```python
from build123d import *

# Parameters (mm, degrees)
EXTRUDE_1_DEPTH     = 15
SKETCH_2_R          = 22.25
EXTRUDE_2_DEPTH     = 560
SKETCH_3_R          = 20
EXTRUDE_3_DEPTH     = 25
SKETCH_4_R          = 4
CUT_EXTRUDE_4_DEPTH = 606.548993339
FILLET_1_R          = 1


with BuildPart() as part:
    # 草图1 → 拉伸1 (new body)
    with BuildSketch(Plane.XY):
        Polygon((37.527767497, 0), (18.763883749, 32.5), (-18.763883749, 32.5), (-37.527767497, 0), (-18.763883749, -32.5), (18.763883749, -32.5), align=None)
    extrude(amount=EXTRUDE_1_DEPTH)

    # 草图2 → 拉伸2 (add)
    with BuildSketch(Plane.XY.offset(15)):
        Circle(SKETCH_2_R)
    extrude(amount=EXTRUDE_2_DEPTH)

    # 草图3 → 拉伸3 (add)
    with BuildSketch(Plane.XY.offset(575)):
        Circle(SKETCH_3_R)
    extrude(amount=EXTRUDE_3_DEPTH)

    # 草图4 → 拉伸4 (cut, through all)
    with BuildSketch(Plane(origin=(-28.145825623, -16.25, 0), x_dir=(0, 0, 1), z_dir=(-0.8660254037844388, -0.4999999999999997, 0))):
        with Locations(Location((587.5, 0, 0), (0, 0, 270))):
            Circle(SKETCH_4_R)
    extrude(amount=-CUT_EXTRUDE_4_DEPTH, mode=Mode.SUBTRACT)

    # 圆角1
    fillet_1_edges = [part.edges().sort_by_distance(p)[0] for p in [
        (0, 32.5, 15),
        (-28.145825623, 16.25, 15),
        (-28.145825623, -16.25, 15),
        (0, -32.5, 15),
        (-22.25, 0, 575),
        (-20, 0, 600),
        (-18.970562748, -6.333857356, 587.5),
        (14.970562748, 13.262060586, 587.5),
        (28.145825623, -16.25, 15),
        (0, -32.5, 0),
        (-28.145825623, -16.25, 0),
        (-28.145825623, 16.25, 0),
        (28.145825623, 16.25, 15),
        (0, 32.5, 0),
        (28.145825623, 16.25, 0),
        (28.145825623, -16.25, 0),
    ]]
    fillet(fillet_1_edges, radius=FILLET_1_R)


solid = part.part
```
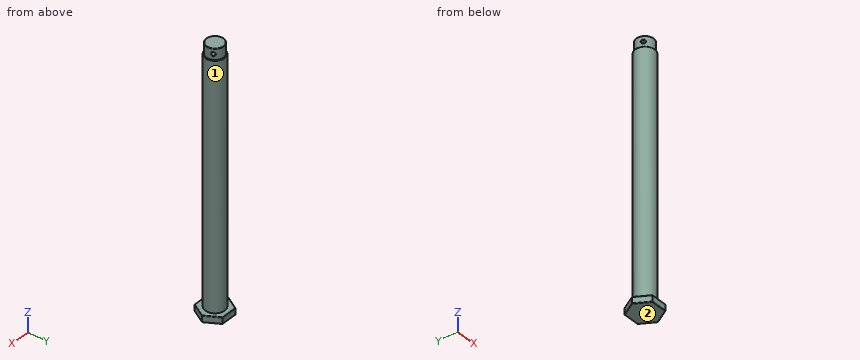
Model file for the job. Use its own axes, mm. Face numbers are marked on the shaded views. A direction names the side the tool comes from. Coordinates: 2 decimals unless noted, no trailing zeros. Loops run counter-clockwise (first coordinate to the right, second up) from the corner with the lowest first, then second, coordinate; pieces in that order, holes last. Notation, with made-up numbers: (-28, 29.5) - (-13, 29.5) arc R16 cw to (-13, 41.5) - close; hole circle Ø9 at (41, 54.5). An arc over 180 degrees is marked (long way). Write item = value, one per line. Start each with the question number.
Item 1: Drop flat-ended pins along their axis: pin 1 Ø3 at (y, z) = (-19, 142.5) entering from +X; pin 2 Ø12 at (x, z) = (-10, 379) entering from +Y; pin 3 Ø2 at (y, z) = (-13.5, 398.5) entering from -X. Give the stop position or say it passes through.
Item 2: Saw through at A-A, the plane z = 536. List the corners of the cut face in (x, y).
Item 3: 3-axis set-ups, long thin cutter, end or side, ignore diameter. For the marked faces 1 and 2: which of +Z, -Z, +X, -X, +Y, -Y reach the whole face in a straight line?
Item 4: Wall check: probe 1 along Z at (x, y) = (-25.5, -6); probe 2 along X at (y, z) = (2, 513); probe 3 along Z at (x, y) = (-14, -10.5). Give the ranges that are in metal, low to high. Write a range as [from, to].
Answers:
q1.pin_1 = 13.74
q1.pin_2 = 21.89
q1.pin_3 = -18.41
q2.outline = circle Ø44.5 at (0, 0)
q3.face_1 = +Z
q3.face_2 = -Z, +X, -X, +Y, -Y
q4.probe_1 = [0, 15]
q4.probe_2 = [-22.16, 22.16]
q4.probe_3 = [0, 584.09], [590.91, 600]
